Here's the drawing with two shaded views (mm, measured from the low corner). I have some questions. A direction names the side the tool comes from. Give positions to 0.01 mm unless a question says otherwise; leave off trailing zeros. Loops run counter-clockwise (first coordinate to the right, second up) from the corner with the lowest first, then second, coordinate; pieces in that order, holes last. Notation, with made-up numbers: M 8.5,58 L 13.5,58 A4 cw 13.5,62 Z; hole C 2.25,-38.75 d2. An arc over 180 degrees is marked long. Put each result on its own line as item: value. Start each with the question number.
1) If we mould it in two halves opening along Y, with no side actions, what happens to the marked faces 4, 5, 6 and 7? For each: +Y half, -Y half, draft (parallel to the pull), parting line (faces both ways), or undercut.
2) Imagine slicing it at B-B (y = 27). Write out the boundary of the cut face in (x, z) (3 decimals), then the cut area to 3 significant figures.
3) Imagine slicing it at A-A (x = 15.25). Write out the boundary of the cut face in (y, z) (3 decimals).
4) Imagine slicing it at C-C (x = 20.75). Write out the boundary of the cut face in (y, z) (3 decimals), then the cut area to 3 significant figures.
5) Please list where these lines run through material, in increasing order: line 1 along Y through (x, z) = (2.25, 0.2) (3 decimals); line 2 along Y through (x, z) = (15, 0.9) (3 decimals); line 3 along X through (y, z) = (13.5, 2.25) (3 decimals). Write a range as from..to.
6) For the marked faces 1, 2 and 3, which set-ups out of +Z, -Z, +X, -X, +Y, -Y let a thin tool reach every point of the face, with its end or its side?
7) For P1, Ø1.6, axis at x = 5, z = 2, coming from the +Y side (3 decimals); P2, Ø1, axis at x = 2, z = 2, coming from the -Y side (3 decimals); P3, Ø1.6, axis at y = 25, z = 2.5, coming from the +X side (3 decimals), each with a flat end and sliding along its axis, tell me the tip position at first contact or that it passes through.
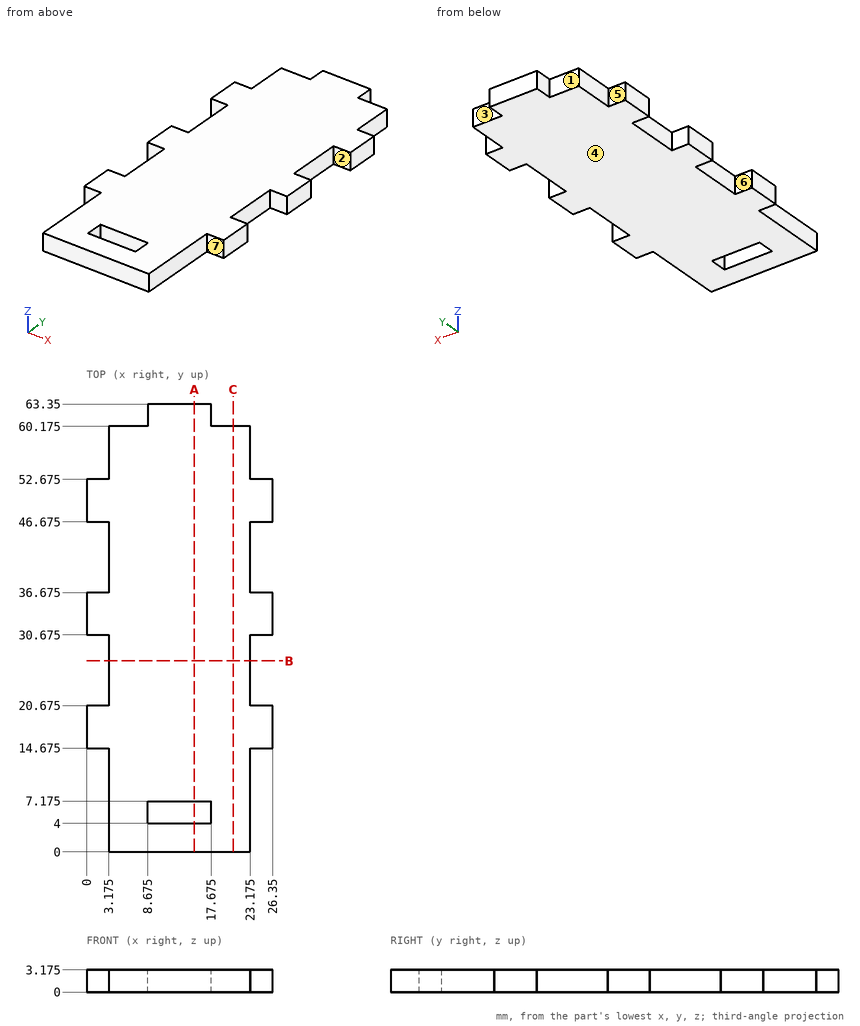
Recorded:
1. face 4: draft
1. face 5: +Y half
1. face 6: undercut
1. face 7: -Y half
2. outline: M 3.175,0 L 23.175,0 L 23.175,3.175 L 3.175,3.175 Z
2. area: 63.5 mm²
3. outline: M 0,0 L 4,0 L 4,3.175 L 0,3.175 Z; M 7.175,0 L 63.35,0 L 63.35,3.175 L 7.175,3.175 Z
4. outline: M 0,0 L 60.175,0 L 60.175,3.175 L 0,3.175 Z
4. area: 191 mm²
5. line 1: 14.675..20.675, 30.675..36.675, 46.675..52.675
5. line 2: 0..4, 7.175..63.35
5. line 3: 3.175..23.175
6. face 1: +Z, -Z, -X, +Y
6. face 2: +Z, -Z, +X
6. face 3: +Z, -Z, +X, +Y
7. P1: y = 60.175
7. P2: y = 14.675
7. P3: x = 23.175
